```python
from build123d import *

# Parameters (mm, degrees)
SKETCH1_W                  = 139.7
SKETCH1_H                  = 127
PLATE_WIDTH_DEPTH          = 6.35
SKETCH2_R                  = 1.6002
SKETCH2_W                  = 77.0509
SKETCH2_H                  = 20.6502
THROUGH_HOLES_DEPTH        = 6.35
SKETCH3_R                  = 6.35
SKETCH3_W                  = 80.2259
SKETCH3_H                  = 23.8252
SKETCH3_W_2                = 77.0509
SKETCH3_H_2                = 20.6502
COVER_CUTOUT_DEPTH         = 2
NUT_INSET_DEPTH            = 1.5875
MATERIAL_REMOVAL_OUTLINE_W = 133.35
MATERIAL_REMOVAL_OUTLINE_H = 120.65
MATERIAL_REMOVAL_OUTLINE_R = 4.7752
MATERIAL_REMOVAL_DEPTH     = 3.175
SKETCH6_W                  = 139.7
SKETCH6_H                  = 127
SKETCH6_W_2                = 133.35
SKETCH6_H_2                = 120.65
BOSS_EXTRUDE1_DEPTH        = 22.098


# Read off the part's stored shape, not the designer's step: Material Removal
with BuildPart() as part:
    # Sketch1 → Plate Width (new body)
    with BuildSketch(Plane.XY):
        Rectangle(SKETCH1_W, SKETCH1_H)
    extrude(amount=PLATE_WIDTH_DEPTH)

    # Sketch2 → Through Holes (cut)
    with BuildSketch(Plane.XY.offset(6.35)):
        with Locations((-51.2699, 46.45025)):
            Circle(SKETCH2_R)
        with Locations((-51.2699, -8.44931)):
            Circle(SKETCH2_R)
        with Locations((50.76952, -8.44931)):
            Circle(SKETCH2_R)
        with Locations((50.76952, 46.45025)):
            Circle(SKETCH2_R)
        with Locations((-0.73025, 26.13025)):
            Rectangle(SKETCH2_W, SKETCH2_H)
    extrude(amount=-THROUGH_HOLES_DEPTH, mode=Mode.SUBTRACT)

    # Sketch3 → Cover Cutout (cut)
    # profile 1 of 4: a face of its own
    with BuildSketch(Plane.XY):
        with Locations((-39.2557, 26.13025)):
            Circle(SKETCH3_R)
    # profile 2 of 4: a face of its own
    with BuildSketch(Plane.XY):
        with Locations((-0.73025, 26.13025)):
            Rectangle(SKETCH3_W, SKETCH3_H)
        with Locations((-0.73025, 26.13025)):
            Rectangle(SKETCH3_W_2, SKETCH3_H_2, mode=Mode.SUBTRACT)
    # profile 3 of 4: a face of its own
    with BuildSketch(Plane.XY):
        with BuildLine():
            Line((-40.8432, 19.981888938), (-40.8432, 32.278611062))
            ThreePointArc((-40.8432, 32.278611062), (-45.6057, 26.13025), (-40.8432, 19.981888938))
        make_face()
    # profile 4 of 4: a face of its own
    with BuildSketch(Plane.XY):
        with BuildLine():
            Line((-39.2557, 19.78025), (-39.2557, 32.48025))
            ThreePointArc((-39.2557, 32.48025), (-40.055827257, 32.429638571), (-40.8432, 32.278611062))
            Line((-40.8432, 32.278611062), (-40.8432, 19.981888938))
            ThreePointArc((-40.8432, 19.981888938), (-40.055827257, 19.830861429), (-39.2557, 19.78025))
        make_face()
    extrude(amount=COVER_CUTOUT_DEPTH, mode=Mode.SUBTRACT)

    # Sketch4 → Nut Inset (cut)
    with BuildSketch(Plane.XY.offset(2)):
        Polygon((-41.514156448, 24.54275), (-40.597612895, 26.13025), (-41.514156448, 27.71775), (-43.347243552, 27.71775), (-44.263787105, 26.13025), (-43.347243552, 24.54275), align=None)
    extrude(amount=NUT_INSET_DEPTH, mode=Mode.SUBTRACT)

    # Material Removal outline → Material Removal (cut)
    with BuildSketch(Plane(origin=(0, 0, 6.35), x_dir=(-1, 0, 0), z_dir=(0, 0, -1))):
        Rectangle(MATERIAL_REMOVAL_OUTLINE_W, MATERIAL_REMOVAL_OUTLINE_H)
        with Locations((-50.76952, -8.44931)):
            Circle(MATERIAL_REMOVAL_OUTLINE_R, mode=Mode.SUBTRACT)
        with Locations((51.2699, -8.44931)):
            Circle(MATERIAL_REMOVAL_OUTLINE_R, mode=Mode.SUBTRACT)
        with Locations((-50.76952, 46.45025)):
            Circle(MATERIAL_REMOVAL_OUTLINE_R, mode=Mode.SUBTRACT)
        with BuildLine():
            Line((42.4307, 39.63035), (42.4307, 33.405088916))
            ThreePointArc((42.4307, 33.405088916), (47.1932, 26.13025), (42.4307, 18.855411084))
            Line((42.4307, 18.855411084), (42.4307, 12.63015))
            Line((42.4307, 12.63015), (-40.9702, 12.63015))
            Line((-40.9702, 12.63015), (-40.9702, 39.63035))
            Line((-40.9702, 39.63035), (42.4307, 39.63035))
        make_face(mode=Mode.SUBTRACT)
        with Locations((51.2699, 46.45025)):
            Circle(MATERIAL_REMOVAL_OUTLINE_R, mode=Mode.SUBTRACT)
    extrude(amount=MATERIAL_REMOVAL_DEPTH, mode=Mode.SUBTRACT)

    # Sketch6 → Boss-Extrude1 (add)
    with BuildSketch(Plane.XY.offset(6.35)):
        Rectangle(SKETCH6_W, SKETCH6_H)
        Rectangle(SKETCH6_W_2, SKETCH6_H_2, mode=Mode.SUBTRACT)
    extrude(amount=BOSS_EXTRUDE1_DEPTH)


solid = part.part
```
Could you check a few things on this model? Use its own coordinates, in mm. A direction names the side the tool comes from. Coordinates: 2 decimals unless noted, no trailing zeros. Loops run counter-clockwise (first coordinate to the right, second up) from the corner with the lowest first, then second, coordinate; pieces in that order, holes last. Notation, with made-up numbers: M 4.5,35.5 L 36.5,35.5 A19 cw 36.5,54.5 Z; hole C 52.5,48 d2. An arc over 180 degrees is marked long. Put each result on its own line as item: value. Start each with the question number.
(1) For faces 1 (the face through (-69.85, -1, 14)), 2 (the face through (-1, 36.455, 4)), 3 (the face through (51, -11, 6.35)), 4 (the face through (69.85, -1, 14)), 5 (the face through (-45.605, 26.247, 0.986)), which set-ups out of +Z, -Z, +X, -X, +Y, -Y let a thin tool reach every point of the face, with its end or its side?
(2) Suppose I cut it at C-C on y = -20. Please give me the cut outline in (x, z) (3 decimals), then the cut area to 3 significant figures.
(3) Thinking about a two-plate mould opening in Y: for faces 6 (the face through (-52.87, -8.38, 3.22)), 7 (the face through (-1, 1, 0)), which applies, pulls with the +Y half, pulls with the -Y half, needs draft (parallel to the pull), parting line crosses it, or undercut?
(4) Suppose I cut it at A-A on x = 33. Please give me the cut outline in (y, z) (3 decimals), then the cut area to 3 significant figures.
(5) I need wall thicknesses on line 1 (Y direction, x = 39.5, z = 4) (3 decimals); line 2 (Y direction, x = -6, z = 6) (3 decimals); line 3 (X direction, y = -31, z = 6.75) (3 decimals). Which ranges of each line are inside material? Lowest first, please. Write a range as from..to.
(6) Suppose I cut it at B-B on z = 20. Please give me the cut outline in (x, y) (3 decimals), then the cut area to 3 significant figures.
(7) Will these pins go through, and if not, where does the flat tip stop? P1, Ø3, axis at x = -38.5, y = -47.5, coming from the +Z side (3 decimals); P2, Ø1.9, axis at x = 50.77, y = -8.45, coming from the +Z side; P3, Ø7.5, axis at x = 49.5, y = 48.5, coming from the +Z side.
Solutions:
1. face 1: +Z, -Z, -X, +Y, -Y
1. face 2: +Z, -Z
1. face 3: +Z
1. face 4: +Z, -Z, +X, +Y, -Y
1. face 5: -Z
2. outline: M -69.85,0 L 69.85,0 L 69.85,28.448 L 66.675,28.448 L 66.675,3.175 L -66.675,3.175 L -66.675,28.448 L -69.85,28.448 Z
2. area: 604 mm2
3. face 6: undercut
3. face 7: needs draft
4. outline: M -63.5,0 L 14.218,0 L 14.218,2 L 15.805,2 L 15.805,6.35 L 12.63,6.35 L 12.63,3.175 L -60.325,3.175 L -60.325,28.448 L -63.5,28.448 Z; M 36.455,2 L 38.043,2 L 38.043,0 L 63.5,0 L 63.5,28.448 L 60.325,28.448 L 60.325,3.175 L 39.63,3.175 L 39.63,6.35 L 36.455,6.35 Z
4. area: 512 mm2
5. line 1: y = -63.5..-60.325, 12.63..39.63, 60.325..63.5
5. line 2: y = -63.5..-60.325, 12.63..15.805, 36.455..39.63, 60.325..63.5
5. line 3: x = -69.85..-66.675, 66.675..69.85
6. outline: M -69.85,-63.5 L 69.85,-63.5 L 69.85,63.5 L -69.85,63.5 Z; hole M -66.675,-60.325 L 66.675,-60.325 L 66.675,60.325 L -66.675,60.325 Z
6. area: 1,650 mm2
7. P1: stops at z = 3.175
7. P2: passes through
7. P3: stops at z = 6.35
